```python
from build123d import *

# Parameters (mm, degrees)
SKETCH_1_W      = 15
SKETCH_1_H      = 1
EXTRUDE_1_DEPTH = 130
SKETCH_3_W      = 1
SKETCH_3_H      = 130
EXTRUDE_2_DEPTH = 14
M3X0_5_1_D      = 2.5


with BuildPart() as part:
    # ｽｹｯﾁ1 → ﾎﾞｽ - 押し出し1 (new body)
    with BuildSketch(Plane(origin=(0, 0, 0), x_dir=(1, 0, 0), z_dir=(0, 1, 0))):
        with Locations((7.5, -0.5)):
            Rectangle(SKETCH_1_W, SKETCH_1_H)
    extrude(amount=EXTRUDE_1_DEPTH)

    # ｽｹｯﾁ3 → ﾎﾞｽ - 押し出し2 (add)
    with BuildSketch(Plane(origin=(0, 0, 0), x_dir=(-1, 0, 0), z_dir=(0, 0, -1))):
        with Locations((-0.5, 65)):
            Rectangle(SKETCH_3_W, SKETCH_3_H)
    extrude(amount=EXTRUDE_2_DEPTH)

    # M3x0.5 ねじ穴1 (through all)
    with Locations(Plane.ZY):
        with Locations((-7, 15), (-7, 75)):
            Hole(M3X0_5_1_D / 2)


solid = part.part
```
Here's how the part is built. I have some questions about the finished solid (model axes, mm). A direction names the side the tool comes from. Round coordinates to 2 decimals unless told otherwise and drop trailing zeros. Write each loop counter-clockwise with the first axis right and the second up, starting at its lowest first coordinate (ties: lowest second). Pieces come first, ordered by that corner, then holes.
Q1. Will these pins go through, and if not, where does the flat tip stop? P1, Ø7, axis at x = 8, y = 72.5, coming from the -Z side; P2, Ø3, axis at y = 75, z = -7, coming from the +X side.
Q2. If we section it at D-D on z = -12: Write out the boundary of the cut face in (x, y).
Q3. If we section it at C-C on y = 117: Write out the boundary of the cut face in (x, z).
Q4. If we mould it in two halves opening along Z, with no side actions, what happens to faces 3 (the flat face through (8, 64, 0)), 4 (the cylindrical face through (0.507, 15.845, -6.079)), 5 (the flat face through (4.2, 130, 0.2))? For each: +Z half, -Z half, draft (parallel to the pull), parting line (faces both ways), or undercut.
Q5. Please list where these lines run through material, in increasing order: probe 1 along Y at (x, z) = (0.5, -7); probe 2 along Z at (x, y) = (7, 10); probe 3 along Z at (x, y) = (0.4, 75).
Q6. If we section it at A-A on z = -7: Write out the boundary of the cut face in (x, y).
Q7. Which directions (+Z, -Z, +X, -X, +Y, -Y) give clear straight access to the entire face, cutting with the end or side of a thin tool? Please do faces 1 (the flat face through (1, 64, -7)), 2 (the cylindrical face through (0.51, 76.24, -6.84)).
Q8. If we section it at B-B on y = 15: Write out the boundary of the cut face in (x, z), plus the area to 3 significant figures.
Answer below:
1. P1: stops at z = 0
1. P2: stops at x = 1
2. outline: (0, 0) - (1, 0) - (1, 130) - (0, 130) - close
3. outline: (0, -14) - (1, -14) - (1, 0) - (15, 0) - (15, 1) - (0, 1) - close
4. face 3: -Z half
4. face 4: undercut
4. face 5: draft
5. probe 1: y = 0 to 13.75, 16.25 to 73.75, 76.25 to 130
5. probe 2: z = 0 to 1
5. probe 3: z = -14 to -8.25, -5.75 to 1
6. outline: (0, 0) - (1, 0) - (1, 13.75) - (0, 13.75) - close; (0, 16.25) - (1, 16.25) - (1, 73.75) - (0, 73.75) - close; (0, 76.25) - (1, 76.25) - (1, 130) - (0, 130) - close
7. face 1: -Z, +X, +Y, -Y
7. face 2: +X, -X
8. outline: (0, -14) - (1, -14) - (1, -8.25) - (0, -8.25) - close; (0, -5.75) - (1, -5.75) - (1, 0) - (15, 0) - (15, 1) - (0, 1) - close
8. area: 26.5 mm2
